Read the model definition and answer for the solid it produces. Units are mm, in the model's axes. Face numbers are marked on the shaded views. A direction names the side the tool comes from. Coordinates: 2 decimals unless noted, no trailing zeros. Loops run counter-clockwise (first coordinate to the right, second up) from the corner with the lowest first, then second, coordinate; pieces in that order, holes last.
Autodesk Inventor part; units mm, degrees
ref_plane "YZ Plane" through (0, 0, 0) normal (1, 0, 0) x (0, 1, 0)
ref_plane "XZ Plane" through (0, 0, 0) normal (0, 1, 0) x (-1, 0, 0)
ref_plane "XY Plane" through (0, 0, 0) normal (0, 0, 1) x (1, 0, 0)
sketch "Skizze1" plane through (0, 0, 0) normal (0, 0, 1) x (1, 0, 0)
  circle A0 centre (0, 0) radius 10
  dimension "d0" = 20
extrude "Extrusion1" add sketch "Skizze1" against normal blind 100
sketch "Skizze2" plane through (0, 0, -100) normal (0, 0, -1) x (-1, 0, 0)
  circle A0 centre (0, 0) radius 10
  circle A1 centre (0, 0) radius 15
  dimension "d3" = 30
extrude "Extrusion2" add sketch "Skizze2" along normal blind 10 contours A0 | A1
sketch "Skizze3" plane through (0, 0, -110) normal (0, 0, -1) x (-1, 0, 0)
  line L0 (10, -5) -> (-10, -5)
  line L1 (-10, -5) -> (-10, 5)
  line L2 (-10, 5) -> (10, 5)
  line L3 (10, 5) -> (10, -5)
  line L4 (10, -5) -> (-10, 5) construction
  line L5 (-10, -5) -> (10, 5) construction
  point P0 (0, 0)
  dimension "d6" = 20
  dimension "d7" = 10
extrude "Extrusion3" add sketch "Skizze3" along normal blind 10
properties part number "Hubstange"
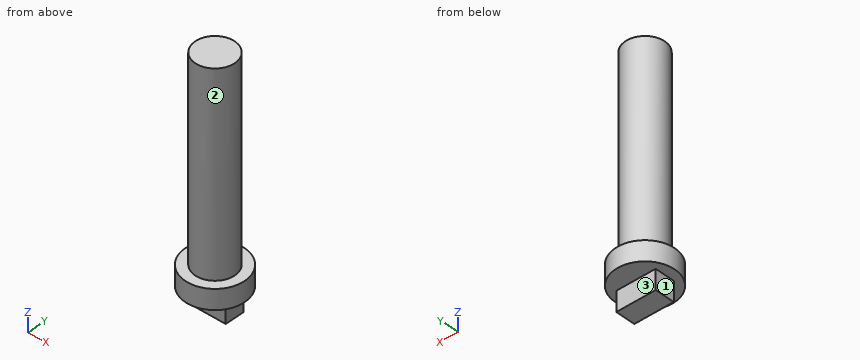
Item 1: Given pin 1 (6 mm diameter, centred on x = 7, z = -54, fed in from +Y); pin 2 (1 mm diameter, centred on x = -8.5, z = -80.5, fed in from +Y); pin 3 (5 mm diameter, centred on x = -10.5, y = -9, fed in from +Z), each flat-ended and moving along its own axis, determine where each tip first touches the part or whether it passes through.
Numbers:
pin 1: stops at y = 9.17
pin 2: stops at y = 6
pin 3: stops at z = -100
Item 2: A cutting plane is placed at D-D on y = -12. Determine the outline of the cut face in (x, z), then the cut area to 3 significant figures.
Numbers:
outline: (-9, -110) - (9, -110) - (9, -100) - (-9, -100) - close
area: 180 mm2
Item 3: Find the intervals of material crossed by line 1 along Z through (x, y) = (3, -11); line 2 along Z through (x, y) = (3, -9); line 3 along Y through (x, z) = (-4.25, -33.5), in increasing order.
Numbers:
line 1: z = -110 to -100
line 2: z = -110 to 0
line 3: y = -9.05 to 9.05
Item 4: A cutting plane is placed at B-B on y = 0. Determine the outline of the cut face in (x, z).
Numbers:
outline: (-15, -110) - (-10, -110) - (-10, -120) - (10, -120) - (10, -110) - (15, -110) - (15, -100) - (10, -100) - (10, 0) - (-10, 0) - (-10, -100) - (-15, -100) - close
Item 5: A cutting plane is placed at A-A on x = 0. Determine the outline of the cut face in (y, z).
Numbers:
outline: (-15, -110) - (-5, -110) - (-5, -120) - (5, -120) - (5, -110) - (15, -110) - (15, -100) - (10, -100) - (10, 0) - (-10, 0) - (-10, -100) - (-15, -100) - close
Item 6: Which of the six approach directions +Z, -Z, +X, -X, +Y, -Y give full straight-line access (tool end or side, diameter ignored) to the marked faces 1, 2 and 3?
Numbers:
face 1: -Z, -X, +Y, -Y
face 2: +Z
face 3: -Z, +X, -X, +Y
Item 7: A cutting plane is placed at C-C on z = -78.5. Determine the outline of the cut face in (x, y).
Numbers:
outline: circle Ø20 at (0, 0)
